```python
from build123d import *

# Parameters (mm, degrees)
SKETCH1_W                       = 200
SKETCH1_H                       = 141.2
BOSS_EXTRUDE1_DEPTH             = 10
SKETCH2_W                       = 100
SKETCH2_H                       = 20.6
BOSS_EXTRUDE2_DEPTH             = 100
FILLET1_R                       = 50
F_10_0MM_DOWEL_HOLE1_D          = 62
F_5_0MM_DOWEL_HOLE1_D           = 5
F_5_0MM_DOWEL_HOLE1_CSINK_D     = 5.05
F_5_0MM_DOWEL_HOLE1_CSINK_ANGLE = 90
FILLET2_R                       = 15


with BuildPart() as part:
    # Sketch1 → Boss-Extrude1 (new body)
    with BuildSketch(Plane(origin=(0, 0, 0), x_dir=(0, 1, 0), z_dir=(0, 0, 1))):
        Rectangle(SKETCH1_W, SKETCH1_H)
    extrude(amount=-BOSS_EXTRUDE1_DEPTH)

    # Sketch2 → Boss-Extrude2 (add)
    with BuildSketch(Plane(origin=(0, 0, 0), x_dir=(0, 1, 0), z_dir=(0, 0, 1))):
        with Locations((0, 60.3)):
            Rectangle(SKETCH2_W, SKETCH2_H)
        with Locations((0, -60.3)):
            Rectangle(SKETCH2_W, SKETCH2_H)
    extrude(amount=BOSS_EXTRUDE2_DEPTH)

    # Fillet1
    fillet1_edges = [part.edges().sort_by_distance(p)[0] for p in [
        (60.3, 50, 100),
        (60.3, -50, 100),
        (-60.3, 50, 100),
        (-60.3, -50, 100),
    ]]
    fillet(fillet1_edges, radius=FILLET1_R - 0.0001)  # a hair under: the kernel refuses the full size

    # Ø10.0mm Dowel Hole1 (through all)
    with Locations(Plane.YZ.offset(70.6)):
        with Locations((0, 50)):
            Hole(F_10_0MM_DOWEL_HOLE1_D / 2)

    # Ø5.0mm Dowel Hole1 (through all)
    with Locations(Plane(origin=(0, 0, 0), x_dir=(0, 1, 0), z_dir=(0, 0, 1))):
        with Locations((75, -37.5), (-75, 37.5), (-75, -37.5), (75, 37.5)):
            CounterSinkHole(F_5_0MM_DOWEL_HOLE1_D / 2, F_5_0MM_DOWEL_HOLE1_CSINK_D / 2, counter_sink_angle=F_5_0MM_DOWEL_HOLE1_CSINK_ANGLE)

    # Fillet2
    fillet2_edges = [part.edges().sort_by_distance(p)[0] for p in [
        (-60.3, -50, 0),
        (-60.3, 50, 0),
        (60.3, -50, 0),
        (60.3, 50, 0),
        (-70.6, -100, -5),
        (-70.6, 100, -5),
        (70.6, 100, -5),
        (70.6, -100, -5),
    ]]
    fillet(fillet2_edges, radius=FILLET2_R)


solid = part.part
```
The listing builds one solid part. Answer for the finished solid, in the listing's coordinates (mm). A direction names the side the tool comes from. Give positions to 0.01 mm unless a question says otherwise; leave off trailing zeros. Write each loop counter-clockwise with the first axis right and the second up, starting at its lowest first coordinate (ties: lowest second). Pieces come first, ordered by that corner, then holes. Notation, with made-up numbers: (-27, -25.5) -> (19, -25.5) arc R16 ccw to (19, -19.5) -> close; hole circle Ø5 at (-37, 32). An arc over 180 degrees is marked (long way). Write item = value, one per line. Start each with the question number.
1) The part is cut by section C-C, the plane z = 62. Determine the outline of the cut face in (x, y), and give its area (3 significant figures).
2) Which of the six approach directions +Z, -Z, +X, -X, +Y, -Y give full straight-line access (tool end or side, diameter ignored) to faces 5 (the face through (60, -50, 32)), 6 (the face through (50, -1, 16)), 7 (the face through (-70.6, 18, 21))?
3) Determine the mould class of faces 1 (the face through (-60.444, 4.036, 80.736)), 2 (the face through (-1, -1, 0)), 3 (the face through (60, 50, 32)), 4 (the face through (60.156, 4.036, 80.736)) for opening direction Y: +Y half, -Y half, draft (parallel to the pull), parting line (faces both ways), or undercut.
4) The part is cut by section A-A, the plane y = -75. Determine the outline of the cut face in (x, z) (3 decimals), and give its area (3 significant figures).
5) Straight lines are drawn through the part: line 1 along Y through (x, z) = (-37.5, -4.25); line 2 along X through (y, z) = (-75, -3); line 3 along X through (y, z) = (-38.5, 16). For each, find the intervals that lie inside material, in ascending order.
6) The part is cut by section D-D, the plane z = 6.5. Determine the outline of the cut face in (x, y), and give its area (3 significant figures).
7) The part is cut by section B-B, the plane x = -37.5. Determine the outline of the cut face in (y, z) (3 decimals), and give its area (3 significant figures).
8) Each of these flat-tipped pins is pushed along its axis until it touches: pin 1 (22.5 mm diameter, centred on x = 61.5, z = 24.5, fed in from +Y); pin 2 (2 mm diameter, centred on y = -29, z = 53.5, fed in from +X); pin 3 (6 mm diameter, centred on x = -37.5, y = 75, fed in from +Z); pin 4 (16.5 mm diameter, centred on x = -63.5, z = 32.5, fed in from -Y). Where does it stop, or does it pass through?
Solutions:
q1.outline = (-70.6, -48.54) -> (-50, -48.54) -> (-50, -28.58) -> (-70.6, -28.58) -> close; (-70.6, 28.58) -> (-50, 28.58) -> (-50, 48.54) -> (-70.6, 48.54) -> close; (50, -48.54) -> (70.6, -48.54) -> (70.6, -28.58) -> (50, -28.58) -> close; (50, 28.58) -> (70.6, 28.58) -> (70.6, 48.54) -> (50, 48.54) -> close
q1.area = 1,640 mm²
q2.face_5 = +Z, +X, -X, -Y
q2.face_6 = +Z, +Y, -Y
q2.face_7 = +Z, -Z, -X, +Y, -Y
q3.face_1 = undercut
q3.face_2 = draft
q3.face_3 = +Y half
q3.face_4 = undercut
q4.outline = (-70.6, -10) -> (-40, -10) -> (-40, -0.025) -> (-40.025, 0) -> (-70.6, 0) -> close; (-35, -10) -> (35, -10) -> (35, -0.025) -> (34.975, 0) -> (-34.975, 0) -> (-35, -0.025) -> close; (40, -10) -> (70.6, -10) -> (70.6, 0) -> (40.025, 0) -> (40, -0.025) -> close
q4.area = 1,310 mm²
q5.line_1 = -100 to -77.5, -72.5 to 72.5, 77.5 to 100
q5.line_2 = -70.6 to -40, -35 to 35, 40 to 70.6
q5.line_3 = -70.6 to -50, 50 to 70.6
q6.outline = (-70.6, -52.64) -> (-50, -52.64) -> (-50, 52.64) -> (-70.6, 52.64) -> close; (50, -52.64) -> (70.6, -52.64) -> (70.6, 52.64) -> (50, 52.64) -> close
q6.area = 4,340 mm²
q7.outline = (-100, -10) -> (-77.5, -10) -> (-77.5, -0.025) -> (-77.525, 0) -> (-100, 0) -> close; (-72.5, -10) -> (72.5, -10) -> (72.5, -0.025) -> (72.475, 0) -> (-72.475, 0) -> (-72.5, -0.025) -> close; (77.5, -10) -> (100, -10) -> (100, 0) -> (77.525, 0) -> (77.5, -0.025) -> close
q7.area = 1,900 mm²
q8.pin_1 = 50.1
q8.pin_2 = through
q8.pin_3 = 0
q8.pin_4 = -50
